from build123d import *
from build123d.topology import SkipClean

# Parameters (mm, degrees)
CROQUIS1_R              = 4.5
CROQUIS1_R_2            = 1.5
SALIENTE_EXTRUIR2_DEPTH = 3
ROSCA1_PITCH            = 0.5
CROQUIS5_W              = 9
CROQUIS5_H              = 5
CROQUIS5_R              = 1.5
SALIENTE_EXTRUIR3_DEPTH = 4
CORTAR_EXTRUIR3_START   = -10
CORTAR_EXTRUIR3_DEPTH   = 10
CROQUIS7_W              = 5
CROQUIS7_H              = 3
CORTAR_EXTRUIR4_DEPTH   = 10
CORTAR_EXTRUIR6_DEPTH   = 10
CROQUIS10_W             = 0.257359313
CROQUIS10_H             = 3.5
CORTAR_EXTRUIR7_DEPTH   = 10


with BuildPart() as part:
    # Croquis1 → Saliente-Extruir2 (new body)
    with BuildSketch(Plane.XY):
        Circle(CROQUIS1_R)
        Circle(CROQUIS1_R_2, mode=Mode.SUBTRACT)
    extrude(amount=SALIENTE_EXTRUIR2_DEPTH)

    # Rosca1: the profile of Perfil de rosca1 profile screwed along a right-hand helix of 6 turns, 6 arcs to a turn; built about Z, then put on its axis
    rosca1_z = Axis((0, 0, 0), (0, 0, 1))
    rosca1_corners = [(1.4997, 0, -0.000173205), (1.770632938, 0, 0.156249999), (1.770632938, 0, 0.218749999), (1.4997, 0, 0.375173204)]
    with BuildLine(mode=Mode.PRIVATE) as rosca1_profile:
        Line(rosca1_corners[0], rosca1_corners[1])
        Line(rosca1_corners[1], rosca1_corners[2])
        Line(rosca1_corners[2], rosca1_corners[3])
        Line(rosca1_corners[3], rosca1_corners[0])
    rosca1_cap = Face(rosca1_profile.wire())
    rosca1_turn_angles = [0, 30, 60, 90, 120, 150, 180, 210, 240, 270, 300, 330, 360]
    rosca1_turn_weights = [1, 0.8660254037844387, 1, 0.8660254037844387, 1, 0.8660254037844387, 1, 0.8660254037844387, 1, 0.8660254037844387, 1, 0.8660254037844387, 1]
    rosca1_turn_rails = [Edge.make_bspline([Vector(p[0], p[1], 0).rotate(rosca1_z, rosca1_turn_angles[k]) / rosca1_turn_weights[k] + Vector(0, 0, p[2] + ROSCA1_PITCH * rosca1_turn_angles[k] / 360) for k in range(13)], [0, 0, 0, 1, 1, 2, 2, 3, 3, 4, 4, 5, 5, 6, 6, 6], 2, rosca1_turn_weights) for p in rosca1_corners]
    rosca1_turn_sides = [Face.make_surface_from_curves(rosca1_turn_rails[p[0]], rosca1_turn_rails[p[1]]) for p in [(0, 1), (1, 2), (2, 3), (3, 0)]]
    rosca1 = Plane(origin=(0, 0, 3), x_dir=(-1, 0, 0), z_dir=(0, 0, -1)) * Solid(Shell([*[p.moved(Location((0, 0, ROSCA1_PITCH * i))) for i in range(6) for p in rosca1_turn_sides], rosca1_cap, rosca1_cap.rotate(rosca1_z, 2160).moved(Location((0, 0, ROSCA1_PITCH * 2160 / 360)))]))
    add(rosca1, mode=Mode.SUBTRACT)

    # Croquis5 → Saliente-Extruir3 (add, symmetric)
    with BuildSketch(Plane(origin=(0, 0, 0), x_dir=(1, 0, 0), z_dir=(0, 1, 0))):
        with Locations((0, 2.5)):
            Rectangle(CROQUIS5_W, CROQUIS5_H)
        with Locations(Location((0, 3, 0), (0, 0, 270))):
            Circle(CROQUIS5_R, mode=Mode.SUBTRACT)
    extrude(amount=SALIENTE_EXTRUIR3_DEPTH, both=True)

    # Croquis6 → Cortar-Extruir3 (cut)
    with SkipClean():  # the faces are left unmerged after this step: merging them gives an invalid solid
        with BuildSketch(Plane.XY.offset(CORTAR_EXTRUIR3_START)):
            with BuildLine():
                Line((-4.5, 4), (-4.5, 0))
                ThreePointArc((-4.5, 0), (-3.842329219, 2.342329219), (-2.061552813, 4))
                Line((-2.061552813, 4), (-4.5, 4))
            make_face()
            with BuildLine():
                Line((4.5, 4), (2.061552813, 4))
                ThreePointArc((2.061552813, 4), (3.842329219, 2.342329219), (4.5, 0))
                Line((4.5, 0), (4.5, 4))
            make_face()
            with BuildLine():
                Line((4.5, -4), (4.5, 0))
                ThreePointArc((4.5, 0), (3.842329219, -2.342329219), (2.061552813, -4))
                Line((2.061552813, -4), (4.5, -4))
            make_face()
            with BuildLine():
                Line((-4.5, 0), (-4.5, -4))
                Line((-4.5, -4), (-2.061552813, -4))
                ThreePointArc((-2.061552813, -4), (-3.842329219, -2.342329219), (-4.5, 0))
            make_face()
        extrude(amount=CORTAR_EXTRUIR3_DEPTH, mode=Mode.SUBTRACT)

    # Croquis7 → Cortar-Extruir4 (cut, symmetric)
    with SkipClean():  # the faces are left unmerged after this step: merging them gives an invalid solid
        with BuildSketch(Plane(origin=(0, 0, 0), x_dir=(0, 0, -1), z_dir=(1, 0, 0))):
            with Locations((2.5, 3)):
                Rectangle(CROQUIS7_W, CROQUIS7_H)
            with Locations((2.5, -3)):
                Rectangle(CROQUIS7_W, CROQUIS7_H)
        extrude(amount=CORTAR_EXTRUIR4_DEPTH, both=True, mode=Mode.SUBTRACT)

    # Croquis9 → Cortar-Extruir6 (cut)
    with SkipClean():  # the faces are left unmerged after this step: merging them gives an invalid solid
        with BuildSketch(Plane(origin=(0, 1.5, 0), x_dir=(1, 0, 0), z_dir=(0, 1, 0))):
            with BuildLine():
                Line((-4.242640687, 0), (-1.892710475, 0))
                ThreePointArc((-1.892710475, 0), (-0.967258097, 0.298907677), (1e-08, 0.4))
                Line((1e-08, 0.4), (-4.242640687, 0.4))
                Line((-4.242640687, 0.4), (-4.242640687, 0))
            make_face()
            with BuildLine():
                Line((-4.5, 0.4), (-4.5, -3))
                ThreePointArc((-4.5, -3), (-3.530819565, -1.20931822), (-1.892710475, 0))
                Line((-1.892710475, 0), (-4.242640687, 0))
                Line((-4.242640687, 0), (-4.242640687, 0.4))
                Line((-4.242640687, 0.4), (-4.5, 0.4))
            make_face()
            with BuildLine():
                ThreePointArc((1e-08, 0.4), (0.967258107, 0.298907675), (1.892710475, 0))
                Line((1.892710475, 0), (4.242640687, 0))
                Line((4.242640687, 0), (4.242640687, 0.4))
                Line((4.242640687, 0.4), (1e-08, 0.4))
            make_face()
            with BuildLine():
                ThreePointArc((1.892710475, 0), (3.530819565, -1.20931822), (4.5, -3))
                Line((4.5, -3), (4.5, 0.4))
                Line((4.5, 0.4), (4.242640687, 0.4))
                Line((4.242640687, 0.4), (4.242640687, 0))
                Line((4.242640687, 0), (1.892710475, 0))
            make_face()
        cortar_extruir6 = extrude(amount=CORTAR_EXTRUIR6_DEPTH, mode=Mode.SUBTRACT)

    # Simetría1: Cortar-Extruir6 across plane
    with SkipClean():  # the faces are left unmerged after this step: merging them gives an invalid solid
        add(cortar_extruir6.mirror(Plane.ZX), mode=Mode.SUBTRACT)

    # Croquis10 → Cortar-Extruir7 (cut)
    with SkipClean():  # the faces are left unmerged after this step: merging them gives an invalid solid
        with BuildSketch(Plane(origin=(0, 1.5, 0), x_dir=(1, 0, 0), z_dir=(0, 1, 0))):
            with BuildLine():
                Line((-4.242640687, 5), (-4.242640687, 1.5))
                Line((-4.242640687, 1.5), (-2.598076211, 1.5))
                ThreePointArc((-2.598076211, 1.5), (-2.984080681, 3.308646222), (-2.236067977, 5))
                Line((-2.236067977, 5), (-4.242640687, 5))
            make_face()
            with BuildLine():
                ThreePointArc((2.236067977, 5), (2.984080681, 3.308646222), (2.598076211, 1.5))
                Line((2.598076211, 1.5), (4.242640687, 1.5))
                Line((4.242640687, 1.5), (4.242640687, 5))
                Line((4.242640687, 5), (2.236067977, 5))
            make_face()
            with Locations((-4.371320344, 3.25)):
                Rectangle(CROQUIS10_W, CROQUIS10_H)
            with Locations((4.371320344, 3.25)):
                Rectangle(CROQUIS10_W, CROQUIS10_H)
        extrude(amount=-CORTAR_EXTRUIR7_DEPTH, mode=Mode.SUBTRACT)


solid = part.part
Verification items for the finished model (mm, model axes). A direction names the side the tool comes from. Give positions to 0.01 mm unless a question says otherwise; leave off trailing zeros. Write each loop counter-clockwise with the first axis right and the second up, starting at its lowest first coordinate (ties: lowest second). Pieces come first, ordered by that corner, then holes.
(1) Cross-section at A-A (z = -3). Enter the section's corners in (x, y).
(2) Material ranges on line 1 (X direction, y = 0.25, z = -3); line 2 (Z direction, x = 0, y = 0.8); line 3 (Z direction, x = 4, y = 1.25), recorded low to high.
(3) Cross-section at D-D (x = -0.5). State how many separate pieces and enclosed holes the cut face has, plus the area to 3 significant figures.
(4) Access from +Z, -Z, +X, -X, +Y, -Y to the whole of each face (thin tool, end or side, straight path). Record for faces 4 (the face through (0, -3, 0)), 5 (the face through (-3.018, 2.486, 0.704)), 6 (the face through (-3.018, -2.486, 0.704)), 7 (the face through (-4, 0, -1.5)).
(5) Mould release check, pull along Y, two halves, no side actions. Record for faces 1 (the face through (0, -2, 3)), 2 (the face through (0, -1.5, -1)), 3 (the face through (0, 0, 0)): +Y half, -Y half, draft (parallel to the pull), parting line (faces both ways), or undercut.
(6) Cross-section at C-C (z = -4.25). Enter the section's corners in (x, y).
(7) Gauge pin test, flat ends, axial feed: pin 1 (2 mm diameter, centred on x = 2, z = 1.5, fed in from +Y); pin 2 (3.5 mm diameter, centred on x = 0, y = 0, fed in from +Z); pin 3 (1.5 mm diameter, centred on y = -2, z = 1.5, fed in from +X); pin 4 (2.5 mm diameter, centred on x = -1, y = -3, fed in from -Z). Record the tip position at first contact, or that the pin passes through.
(8) Cross-section at B-B (x = 2.75). Enter the section's corners in (y, z), plus the area to 3 significant figures.
Worked out:
1. outline: (-3, -1.5) - (-1.5, -1.5) - (-1.5, 1.5) - (-3, 1.5) - close; (1.5, -1.5) - (3, -1.5) - (3, 1.5) - (1.5, 1.5) - close
2. line 1: x = -3 to -1.5, 1.5 to 3
2. line 2: z = -5 to -4.5, -1.5 to 0
2. line 3: z = -1.5 to 3
3. separate pieces: 3
3. enclosed holes: 0
3. area: 24.2 mm2
4. face 4: -Z, +X, -X, -Y
4. face 5: -Z, -X, +Y
4. face 6: -Z, -X, -Y
4. face 7: -X, +Y, -Y
5. face 1: draft
5. face 2: -Y half
5. face 3: undercut
6. outline: (-2.73, -1.5) - (-0.83, -1.5) - (-0.83, 1.5) - (-2.73, 1.5) - close; (0.83, -1.5) - (2.73, -1.5) - (2.73, 1.5) - (0.83, 1.5) - close
7. pin 1: stops at y = 4.39
7. pin 2: stops at z = 3
7. pin 3: stops at x = 4.32
7. pin 4: stops at z = 0
8. outline: (-3.56, 0.49) - (-1.5, 0.49) - (-1.5, -1.5) - (1.5, -1.5) - (1.5, 0.49) - (3.56, 0.49) - (3.56, 3) - (-3.56, 3) - close; (-1.5, -4.2) - (1.5, -4.2) - (1.5, -1.8) - (-1.5, -1.8) - close
8. area: 31.0 mm2
